Can you work these out from the model? Positions are in its coordinate system, mm. Give positions to 0.01 mm unless a question says otherwise; leave off trailing zeros. Order: outer loops, then holes, each group sorted by start corner. A loop starts at its lowest first (then second) coordinate and runs counter-clockwise, first axis right, second up. Notation, with made-up numbers: M 10.25,30.5 L 67.25,30.5 A16 cw 67.25,53.5 Z; hole C 57,82 d6. An arc over 180 degrees is marked long. One line per question, with ' | ' between items. Start each with the question number.
1) If we section it at C-C, the plane y = 45: Please give me the cut outline in (x, z).
2) Please list where these lines run through material, in increasing order: line 1 along Y through (x, z) = (142.5, 3.25); line 2 along Y through (x, z) = (255.5, -1.25); line 3 along X through (y, z) = (27, 3). Write a range as [from, to].
3) If we section it at A-A, the plane z = -2.75: Please give me the cut outline in (x, y), plus the area to 3 significant figures.
4) I'm going to push flat-ended pins straight in: pin 1 Ø1.5 at (x, z) = (177, 2.5) entering from -Y; pin 2 Ø4 at (x, z) = (250.5, 2.5) entering from +Y. Where does each tip first touch, or does it pass through?
5) If we section it at B-B, the plane x = 172: Please give me the cut outline in (y, z).
Autodesk Inventor part; units mm, degrees
ref_plane "YZ Plane" through (0, 0, 0) normal (1, 0, 0) x (0, 1, 0)
ref_plane "XZ Plane" through (0, 0, 0) normal (0, 1, 0) x (-1, 0, 0)
ref_plane "XY Plane" through (0, 0, 0) normal (0, 0, 1) x (1, 0, 0)
sketch "Sketch3" plane through (0, 0, 0) normal (0, 0, 1) x (1, 0, 0)
  line L0 (0, 0) -> (300, 0)
  line L1 (300, 0) -> (300, 30)
  line L2 (300, 30) -> (-5.542, 53.9641)
  line L3 (45, 50) -> (45, 0)
  dimension "d11" = 300
  dimension "d12" = 30
  dimension "d13" = 45
  dimension "d14" = 50
extrude "Plate1" add sketch "Sketch3" along normal mid plane 8
fillet "Corner Round1" radius 6 1 edges at (300, 30, 0)
equation "\"d15\" = Thickness"
equation "\"BendRadius\" = Thickness"
equation "\"BendReliefWidth\" = Thickness"
equation "\"BendReliefDepth\" = 0.5 * Thickness"
equation "\"CornerReliefSize\" = 4 * Thickness"
equation "\"MinimumRemnant\" = 2 * Thickness"
equation "\"TransitionRadius\" = BendRadius"
equation "\"JacobiRadiusSize\" = BendRadius"
equation "\"GapSize\" = Thickness"
properties part number "PNS-725 charging hatch reinf D1200" material "Steel"
Results found:
1) outline: M 45,-4 L 108.75,-4 L 108.75,4 L 45,4 Z
2) line 1: y = [0, 42.35] | line 2: y = [0, 33.49] | line 3: x = [45, 299.43]
3) outline: M 45,0 L 300,0 L 300,24.45 A6 ccw 294.47,30.43 L 45,50 Z | area: 10,200 mm²
4) pin 1: stops at y = 0 | pin 2: stops at y = 34.04
5) outline: M 0,-4 L 40.04,-4 L 40.04,4 L 0,4 Z
